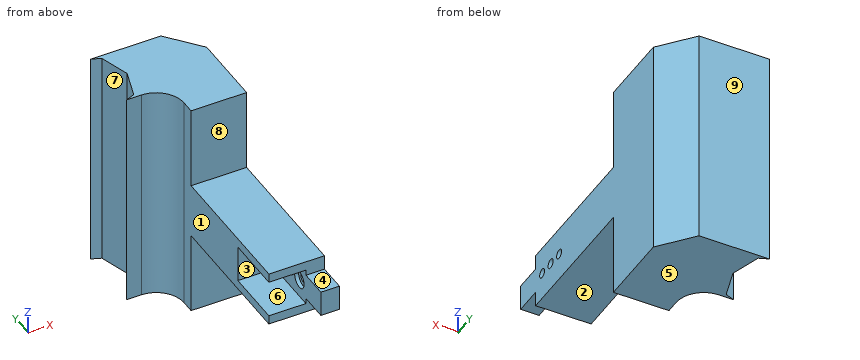
Autodesk Inventor part; units mm, degrees
ref_plane "Work Plane1" through (0, 0, -15) normal (0, 0, 1) x (1, 0, 0)
ref_plane "YZ Plane" through (0, 0, 0) normal (1, 0, 0) x (0, 1, 0)
ref_plane "XZ Plane" through (0, 0, 0) normal (0, 1, 0) x (-1, 0, 0)
sketch "Sketch1" plane through (0, 0, 0) normal (0, 0, 1) x (1, 0, 0)
  line L0 (0, 0) -> (25, 0)
  line L1 (25, 0) -> (25, 40)
  line L2 (25, 40) -> (0, 40)
  line L3 (0, 40) -> (0, 0)
  dimension "d1" = 25
  dimension "d2" = 40
  dimension "d3" = 25
extrude "Extrusion1" add sketch "Sketch1" against normal blind 30
sketch "Sketch2" plane through (25, 0, 0) normal (1, 0, 0) x (0, 0, -1)
  line L0 (0, 0) -> (30, 0)
  circle A0 centre (15, 6.56) radius 2.46
extrude "Extrusion2" cut sketch "Sketch2" against normal blind 30
sketch "Sketch3" plane through (0, 0, 0) normal (-1, 0, 0) x (0, 0, 1)
  line L0 (0, 0) -> (-30, 0)
  line L1 (-25.05, 0) -> (-4.95, 0)
  line L2 (-4.95, 0) -> (-4.95, 33.12)
  line L3 (-4.95, 33.12) -> (-25.05, 33.12)
  line L4 (-25.05, 33.12) -> (-25.05, 0)
  dimension "d11" = 20.1
extrude "Extrusion3" cut sketch "Sketch3" against normal blind 20
sketch "Sketch4" plane through (0, 0, 0) normal (0, -1, 0) x (1, 0, 0)
  line L0 (20, -4.95) -> (20, -25.05)
  line L1 (20, -15) -> (25, -15)
  line L2 (25, 0) -> (25, -30)
  line L3 (20, -8.025) -> (25, -8.025)
  line L4 (25, -8.025) -> (25, -21.975)
  line L5 (25, -21.975) -> (20, -21.975)
  line L6 (20, -21.975) -> (20, -8.025)
  line L7 (20, -8.025) -> (25, -21.975) construction
  line L8 (25, -8.025) -> (20, -21.975) construction
  line L9 (25, -12.54) -> (25, -17.46)
  point P0 (0, 0)
  point P1 (22.5, -15)
  dimension "d14" = 13.95
extrude "Extrusion4" add sketch "Sketch4" along normal blind 15
sketch "Sketch5" plane through (20, 0, 0) normal (-1, 0, 0) x (0, 0, 1)
  circle A0 centre (-15, 6.56) radius 2.46
  circle A1 centre (-15, 6.56) radius 4.7025
  circle A2 centre (-15, 6.56) radius 2.46
  circle A3 centre (-15, 6.56) radius 2.46
  point P0 (0, 0)
  dimension "d17" = 9.405
extrude "Extrusion5" cut sketch "Sketch5" against normal blind 2.1
sketch "Sketch6" plane through (25, 0, 0) normal (1, 0, 0) x (0, 0, -1)
  circle A0 centre (15, 6.56) radius 4.7025
  line L0 (15, 6.56) -> (15, 23.56)
  circle A1 centre (15, 23.56) radius 2.46
  point P0 (0, 0)
  dimension "d20" = 17
  dimension "d21" = 4.92
extrude "Extrusion6" cut sketch "Sketch6" against normal blind 10 contours A1
sketch "Sketch7" plane through (20, 0, 0) normal (-1, 0, 0) x (0, 0, 1)
  circle A0 centre (-15, 23.56) radius 2.46
  circle A1 centre (-15, 23.56) radius 4.7025
  point P0 (0, 0)
  dimension "d24" = 9.405
extrude "Extrusion7" cut sketch "Sketch7" against normal blind 2.1
sketch "Sketch9" plane through (25, 0, 0) normal (1, 0, 0) x (0, 0, -1)
  circle A0 centre (15, 6.56) radius 2.46
  circle A1 centre (15, 6.56) radius 2.46
  circle A2 centre (15, 23.56) radius 2.46
  circle A3 centre (15, 23.56) radius 2.46
  line L0 (30, 40) -> (30, 0)
  line L1 (30, 0) -> (30, 40)
  line L2 (30, 40) -> (0, 40)
  line L3 (0, 40) -> (0, 0)
  line L4 (0, 0) -> (8.025, 0)
  line L5 (21.975, 0) -> (21.975, -15)
  line L6 (21.975, -15) -> (8.025, -15)
  line L7 (8.025, -15) -> (8.025, 0)
  line L8 (0, 0) -> (8.025, 0)
  line L9 (21.975, 0) -> (30, 0)
extrude "Extrusion8" add sketch "Sketch9" along normal blind 5
sketch "Sketch10" plane through (0, 40, 0) normal (0, 1, 0) x (1, 0, 0)
  line L0 (0, 30) -> (30, 30)
  line L1 (30, 0) -> (0, 0)
  line L2 (0, 30) -> (30, 30)
  line L3 (30, 30) -> (30, 0)
  line L4 (30, 0) -> (0, 0)
  line L5 (0, 0) -> (0, 30)
extrude "Extrusion9" add sketch "Sketch10" along normal blind 30
sketch "Sketch12" plane through (30, 0, 0) normal (1, 0, 0) x (0, 0, -1)
  circle A0 centre (15, 6.56) radius 2.46
  line L0 (15, 6.56) -> (15, 15.06)
  circle A1 centre (15, 15.06) radius 2.525
  point P0 (0, 0)
  dimension "d31" = 8.5
  dimension "d33" = 5.05
extrude "Extrusion10" cut sketch "Sketch12" against normal blind 30 contours A1
sketch "Sketch14" plane through (0, 0, 0) normal (0, 0, 1) x (1, 0, 0)
  line L0 (30, 70) -> (0, 70)
  line L1 (0, 70) -> (0, 85)
  line L2 (-15, 100) -> (-23, 100)
  line L3 (30, 0) -> (30, 70)
  line L4 (30, 118) -> (30, 70)
  arc A0 (0, 85) -> (-15, 100) centre (-15, 85) ccw
  line L5 (30, 105) -> (30, 100)
  line L6 (-18, 134) -> (-23, 136)
  line L7 (-18, 102) -> (-23, 100)
  line L8 (-18, 102) -> (-13, 118)
  line L9 (-13, 118) -> (-18, 134)
  line L10 (15, 136) -> (30, 118)
  line L11 (-23, 136) -> (15, 136)
  point P0 (0, 0)
  point P1 (0, 100)
  dimension "d47" = 30
  dimension "d54" = 15
extrude "Extrusion12" add sketch "Sketch14" against normal blind 30
sketch "Sketch15" plane through (0, 0, -25.05) normal (-1, 0, 0) x (0, 0, 1)
  line L0 (0, 33.12) -> (20.1, 33.12)
  line L1 (20.1, 33.12) -> (20.1, 0)
  line L2 (0, 33.12) -> (20.1, 33.12)
  line L3 (20.1, 33.12) -> (20.1, 31.1)
  line L4 (20.1, 31.1) -> (0, 31.1)
  line L5 (0, 31.1) -> (0, 33.12)
  point P0 (25.05, 0)
  dimension "d57" = 2.02
extrude "Extrusion13" add sketch "Sketch15" against normal blind 20
sketch "Sketch22" plane through (0, 0, 0) normal (0, 0, 1) x (1, 0, 0)
  line L0 (-15, 100) -> (-23, 100)
  line L1 (-15, 100) -> (-23, 100)
  line L2 (-23, 100) -> (-18, 102)
  line L3 (-23, 100) -> (-18, 102)
  line L4 (-18, 102) -> (-13, 118)
  line L5 (-18, 102) -> (-13, 118)
  line L6 (-13, 118) -> (-18, 134)
  line L7 (-13, 118) -> (-18, 134)
  line L8 (-18, 134) -> (-23, 136)
  line L9 (-18, 134) -> (-23, 136)
  line L10 (-23, 136) -> (15, 136)
  line L11 (-23, 136) -> (15, 136)
  line L12 (15, 136) -> (30, 118)
  line L13 (15, 136) -> (30, 118)
  line L14 (30, 118) -> (30, 78)
  line L15 (30, 0) -> (30, 118)
  line L16 (30, 78) -> (0, 78)
  arc A0 (0, 85) -> (-15, 100) centre (-15, 85) ccw
  line L17 (0, 78) -> (0, 85)
  arc A1 (0, 85) -> (-15, 100) centre (-15, 85) ccw
  point P0 (0, 0)
  dimension "d82" = 40
extrude "Extrusion14" add sketch "Sketch22" along normal blind 45
ref_plane "Work Plane1" through (0, 0, -15) normal (0, 0, 1) x (1, 0, 0)
mirror "Mirror1" about plane through (0, 0, -15) normal (0, 0, 1) of "Extrusion14"
properties part number "rec_a_32mm_x_120mm"
Read the model definition and answer for the solid it produces. Units are mm, in the model's axes. Face numbers are marked on the shaded views. A direction names the side the tool comes from. Round coordinates to 2 decimals unless told otherwise and drop trailing zeros. Loops run counter-clockwise (first coordinate to the right, second up) from the corner with the lowest first, then second, coordinate; pieces in that order, holes last.
Q1. Section D-D on z = -50 is taken. Write down the section's boundary in (x, y).
Q2. Section B-B on y = 23.56 is taken. Write down the section's boundary in (x, z).
Q3. Section C-C on x = 5.5 is taken. Write down the section's boundary in (y, z), and give its area (3 significant figures).
Q4. Which of the six approach directions +Z, -Z, +X, -X, +Y, -Y give full straight-line access (tool end or side, diameter ignored) to the marked faces 1, 2, 3, 4 and 5?
Q5. Determine the mould class of the marked faces 6, 7, 8 and 9 for opening direction Y: released by +Y, released by -Y, zero draft, split by the parting line, or undercut.
Q6. Consider probe 1 along Y at (x, z) = (27, -15) (3 decimals); probe 2 along Y at (x, z) = (24.5, -15) (3 decimals); probe 3 along Y at (x, z) = (14, -45). Determine where each line is inside the solid, lowest interval first.
Q7. Section A-A on z = -15 is taken. Give the number of separate pieces and of enclosed holes in the cut face, and give its area (3 significant figures).
Q8. Each of these flat-tipped pins is pushed along its axis until it touches: pin 1 (22 mm diameter, centred on x = 7, z = -15.5, fed in from -Y); pin 2 (1.5 mm diameter, centred on x = 1, z = -10, fed in from -Y); pin 3 (16 mm diameter, centred on x = 14.5, y = 9, fed in from -Z). Where does it stop, or does it pass through?
Output:
1. outline: (-23, 100) - (-15, 100) arc R15 cw to (0, 85) - (0, 78) - (30, 78) - (30, 118) - (15, 136) - (-23, 136) - (-18, 134) - (-13, 118) - (-18, 102) - close
2. outline: (0, -30) - (30, -30) - (30, -17.46) - (22.1, -17.46) - (22.1, -19.7) - (20, -19.7) - (20, -25.05) - (0, -25.05) - close; (0, -4.95) - (20, -4.95) - (20, -10.3) - (22.1, -10.3) - (22.1, -12.54) - (30, -12.54) - (30, 0) - (0, 0) - close
3. outline: (0, -30) - (78, -30) - (78, -75) - (136, -75) - (136, 45) - (78, 45) - (78, 0) - (0, 0) - (0, -4.95) - (31.1, -4.95) - (31.1, -25.05) - (0, -25.05) - close
3. area: 8,670 mm2
4. face 1: +Z, -Z, -X, -Y
4. face 2: -Z, +X, -X, -Y
4. face 3: -X, -Y
4. face 4: +Z, +X, -X, -Y
4. face 5: -Z, +X, -X, +Y, -Y
5. face 6: zero draft
5. face 7: undercut
5. face 8: released by -Y
5. face 9: released by +Y
6. probe 1: y = -15 to 4.1, 9.02 to 12.535, 17.585 to 21.1, 26.02 to 121.6
6. probe 2: y = -15 to 4.1, 9.02 to 12.535, 17.585 to 21.1, 26.02 to 124.6
6. probe 3: y = 78 to 136
7. separate pieces: 4
7. enclosed holes: 0
7. area: 3,930 mm2
8. pin 1: stops at y = 0
8. pin 2: stops at y = 31.1
8. pin 3: stops at z = -30
